```python
from build123d import *

# Parameters (mm, degrees)
SKETCH_1_W               = 17
SKETCH_1_H               = 40
EXTRUDE_1_DEPTH          = 50
SKETCH_2_W               = 17
SKETCH_2_H               = 1
CUT_EXTRUDE_1_DEPTH      = 67.2495283
SKETCH_4_W               = 0.5
SKETCH_4_H               = 39
EXTRUDE_2_DEPTH          = 50
SKETCH_5_R               = 15.5
CUT_EXTRUDE_2_DEPTH      = 17.5
CUT_EXTRUDE_3_DEPTH      = 17.5
CUT_EXTRUDE_4_DEPTH      = 3
CUT_EXTRUDE_START        = -64
CUT_EXTRUDE_7_DEPTH      = 64
SKETCH_9_W               = 5
SKETCH_9_H               = 3
EXTRUDE_3_DEPTH          = 17.5
CUT_EXTRUDE_8_DEPTH      = 54.087192429
CUT_EXTRUDE_8_DEPTH_BACK = 54.087192429
CUT_EXTRUDE_9_DEPTH      = 64


with BuildPart() as part:
    # 草图1 → 凸台-拉伸1 (new body)
    with BuildSketch(Plane(origin=(0, 0, 0), x_dir=(1, 0, 0), z_dir=(0, 1, 0))):
        with Locations((8.5, -20)):
            Rectangle(SKETCH_1_W, SKETCH_1_H)
    extrude(amount=EXTRUDE_1_DEPTH)

    # 草图2 → 切除-拉伸1 (cut, through all)
    with BuildSketch(Plane.XZ):
        with Locations((8.5, 39.5)):
            Rectangle(SKETCH_2_W, SKETCH_2_H)
    extrude(amount=-CUT_EXTRUDE_1_DEPTH, mode=Mode.SUBTRACT)

    # 草图4 → 凸台-拉伸2 (add)
    with BuildSketch(Plane.XZ):
        with Locations((-0.25, 19.5)):
            Rectangle(SKETCH_4_W, SKETCH_4_H)
    extrude(amount=-EXTRUDE_2_DEPTH)

    # 草图5 → 切除-拉伸2 (cut)
    with BuildSketch(Plane(origin=(17, 0, 0), x_dir=(0, 0, -1), z_dir=(1, 0, 0))):
        with Locations((-22, 4.5)):
            Circle(SKETCH_5_R)
    extrude(amount=-CUT_EXTRUDE_2_DEPTH, mode=Mode.SUBTRACT)

    # 草图6 → 切除-拉伸3 (cut)
    with BuildSketch(Plane(origin=(17, 0, 0), x_dir=(0, 0, -1), z_dir=(1, 0, 0))):
        Polygon((0, 3), (0, 24), (0, 50), (-39, 50), (-39, 24), (-22, 24), (-5, 24), (-5, 3), align=None)
    extrude(amount=-CUT_EXTRUDE_3_DEPTH, mode=Mode.SUBTRACT)

    # 草图7 → 切除-拉伸4 (cut)
    with BuildSketch(Plane(origin=(0, 3, 0), x_dir=(1, 0, 0), z_dir=(0, 1, 0))):
        with BuildLine():
            ThreePointArc((8.25, -0.9), (6.65, -2.5), (8.25, -4.1))
            Line((8.25, -4.1), (8.25, -0.9))
        make_face()
        with BuildLine():
            Line((8.25, -0.9), (8.25, -4.1))
            ThreePointArc((8.25, -4.1), (9.38137085, -3.63137085), (9.85, -2.5))
            ThreePointArc((9.85, -2.5), (9.38137085, -1.36862915), (8.25, -0.9))
        make_face()
    extrude(amount=-CUT_EXTRUDE_4_DEPTH, mode=Mode.SUBTRACT)

    # 草图8 → 切除-拉伸7 (cut)
    with BuildSketch(Plane.ZY.offset(0.5).offset(CUT_EXTRUDE_START)):
        with BuildLine():
            Line((5, 3), (5, 4.5))
            Line((5, 4.5), (-8.613521725, 4.5))
            Line((-8.613521725, 4.5), (17.256515703, -28.446816898))
            Line((17.256515703, -28.446816898), (39, 0))
            Line((39, 0), (36.832396974, 0))
            ThreePointArc((36.832396974, 0), (22, -11), (7.167603026, 0))
            Line((7.167603026, 0), (0, 0))
            Line((0, 0), (0, 3))
            Line((0, 3), (5, 3))
        make_face()
        with BuildLine():
            ThreePointArc((7.167603026, 0), (6.667809141, 2.225373998), (6.5, 4.5))
            Line((6.5, 4.5), (5, 4.5))
            Line((5, 4.5), (5, 3))
            Line((5, 3), (0, 3))
            Line((0, 3), (0, 0))
            Line((0, 0), (7.167603026, 0))
        make_face()
        with BuildLine():
            Line((37.5, 4.5), (22, 4.5))
            Line((22, 4.5), (6.5, 4.5))
            ThreePointArc((6.5, 4.5), (6.667809141, 2.225373998), (7.167603026, 0))
            ThreePointArc((7.167603026, 0), (22, -11), (36.832396974, 0))
            ThreePointArc((36.832396974, 0), (37.332190859, 2.225373998), (37.5, 4.5))
        make_face()
        with BuildLine():
            Line((6.5, 4.5), (22, 4.5))
            Line((22, 4.5), (37.5, 4.5))
            ThreePointArc((37.5, 4.5), (22, 20), (6.5, 4.5))
        make_face()
        with BuildLine():
            Line((39, 4.5), (37.5, 4.5))
            ThreePointArc((37.5, 4.5), (37.332190859, 2.225373998), (36.832396974, 0))
            Line((36.832396974, 0), (39, 0))
            Line((39, 0), (39, 4.5))
        make_face()
    extrude(amount=CUT_EXTRUDE_7_DEPTH, mode=Mode.SUBTRACT)

    # 草图9 → 凸台-拉伸3 (add)
    with BuildSketch(Plane.ZY.offset(0.5)):
        with Locations((2.5, 6)):
            Rectangle(SKETCH_9_W, SKETCH_9_H)
        with Locations((41.5, 6)):
            Rectangle(SKETCH_9_W, SKETCH_9_H)
    extrude(amount=-EXTRUDE_3_DEPTH)

    # 草图10 → 切除-拉伸8 (cut, two sides: drawn at the far end of the back side and taken through both)
    with BuildSketch(Plane.ZY.offset(0.5).offset(-CUT_EXTRUDE_8_DEPTH_BACK)):
        with BuildLine():
            Line((5, 24), (5, 14.052486587))
            ThreePointArc((5, 14.052486587), (12.151738439, 21.330381583), (22, 24))
            Line((22, 24), (5, 24))
        make_face()
        with BuildLine():
            Line((39, 24), (22, 24))
            ThreePointArc((22, 24), (31.848261561, 21.330381583), (39, 14.052486587))
            Line((39, 14.052486587), (39, 24))
        make_face()
    extrude(amount=CUT_EXTRUDE_8_DEPTH + CUT_EXTRUDE_8_DEPTH_BACK, mode=Mode.SUBTRACT)

    # 草图11 → 切除-拉伸9 (cut)
    with BuildSketch(Plane(origin=(0, 7.5, 0), x_dir=(1, 0, 0), z_dir=(0, 1, 0))):
        with BuildLine():
            ThreePointArc((8.25, -0.9), (6.65, -2.5), (8.25, -4.1))
            Line((8.25, -4.1), (8.25, -0.9))
        make_face()
        with BuildLine():
            Line((8.25, -0.9), (8.25, -4.1))
            ThreePointArc((8.25, -4.1), (9.38137085, -3.63137085), (9.85, -2.5))
            ThreePointArc((9.85, -2.5), (9.38137085, -1.36862915), (8.25, -0.9))
        make_face()
        with BuildLine():
            ThreePointArc((9.85, -41.5), (9.38137085, -40.36862915), (8.25, -39.9))
            Line((8.25, -39.9), (8.25, -43.1))
            ThreePointArc((8.25, -43.1), (9.38137085, -42.63137085), (9.85, -41.5))
        make_face()
        with BuildLine():
            Line((8.25, -43.1), (8.25, -39.9))
            ThreePointArc((8.25, -39.9), (6.65, -41.5), (8.25, -43.1))
        make_face()
    extrude(amount=-CUT_EXTRUDE_9_DEPTH, mode=Mode.SUBTRACT)


solid = part.part
```
The listing builds one solid part. Answer for the finished solid, in the listing's coordinates (mm). A direction names the side the tool comes from. Round coordinates to 2 decimals unless told otherwise and drop trailing zeros. Order: outer loops, then holes, each group sorted by start corner. A loop starts at its lowest first (then second) coordinate and runs counter-clockwise, first axis right, second up. Notation, with made-up numbers: (79.25, 62.25) -> (136.25, 62.25) arc R16 cw to (136.25, 66.25) -> close; hole circle Ø11 at (-7, 76). An arc over 180 degrees is marked (long way). Answer as CSV lines item,"result".
Q1. Which of the six approach directions +Z, -Z, +X, -X, +Y, -Y give full straight-line access (tool end or side, diameter ignored) to faces 4 (the flat face through (8, 11, 5)), 5 (the flat face through (17, 20.1, 23.5)), 6 (the flat face through (8, 11, 39))?
Computed values:
face 4,"-Z, +X, -X, +Y"
face 5,"+Z, -Z, +X, +Y, -Y"
face 6,"+Z, +X, -X, +Y"
Q2. A cutting plane is placed at B-B on x = 5.5. Determine the outline of the cut face in (y, z).
Computed values:
outline,"(4.5, 0) -> (7.5, 0) -> (7.5, 5) -> (14.05, 5) arc R19.5 ccw to (14.05, 39) -> (7.5, 39) -> (7.5, 44) -> (4.5, 44) -> (4.5, 37.5) arc R15.5 cw to (4.5, 6.5) -> close"
Q3. A cutting plane is placed at C-C on z = 32. Determine the outline of the cut face in (x, y).
Computed values:
outline,"(-0.5, 16.34) -> (17, 16.34) -> (17, 21.24) -> (-0.5, 21.24) -> close"
Q4. For a pull along Y with two mould halves and no side action, classify faces 1 (the flat face through (10, 7.5, 41)), 2 (the cylindrical face through (8, 20, 22)), 3 (the flat face through (8, 6, 44)) as +Y half, -Y half, draft (parallel to the pull), parting line (faces both ways), or undercut.
Computed values:
face 1,"+Y half"
face 2,"-Y half"
face 3,"draft"
Q5. A cutting plane is placed at D-D on y = 11. Determine the outline of the cut face in (x, z), plus the area to 3 significant figures.
Computed values:
outline,"(-0.5, 5) -> (17, 5) -> (17, 7.93) -> (-0.5, 7.93) -> close; (-0.5, 36.07) -> (17, 36.07) -> (17, 39) -> (-0.5, 39) -> close"
area,"103 mm^2"
Q6. A cutting plane is placed at A-A on y = 18.5. Determine the outline of the cut face in (x, z), plus the area to 3 significant figures.
Computed values:
outline,"(-0.5, 8.43) -> (17, 8.43) -> (17, 15.35) -> (-0.5, 15.35) -> close; (-0.5, 28.65) -> (17, 28.65) -> (17, 35.57) -> (-0.5, 35.57) -> close"
area,"242 mm^2"
Q7. Given pin 1 (2 mm diameter, centred on x = 13.5, z = 20, fed in from -Y); pin 2 (7 mm diameter, centred on x = 7.5, y = 12, fed in from -Z); pin 3 (1.5 mm diameter, centred on x = 9.5, z = 40.5, fed in from +Y), each flat-ended and moving along its own axis, determine where each tip first touches the part or whether it passes through.
Computed values:
pin 1,"stops at y = 19.71"
pin 2,"stops at z = 5"
pin 3,"stops at y = 7.5"
Q8. Consider line 1 (Z direction, x = 16.25, y = 5.5); line 2 (Z direction, x = 12, y = 18.5); line 3 (Y direction, x = 10.25, z = 24). Determine where each line is inside the solid, lowest interval first. Write a range as from..to.
Computed values:
line 1,"z = 0..6.53, 37.47..44"
line 2,"z = 8.43..15.35, 28.65..35.57"
line 3,"y = 19.87..23.9"
